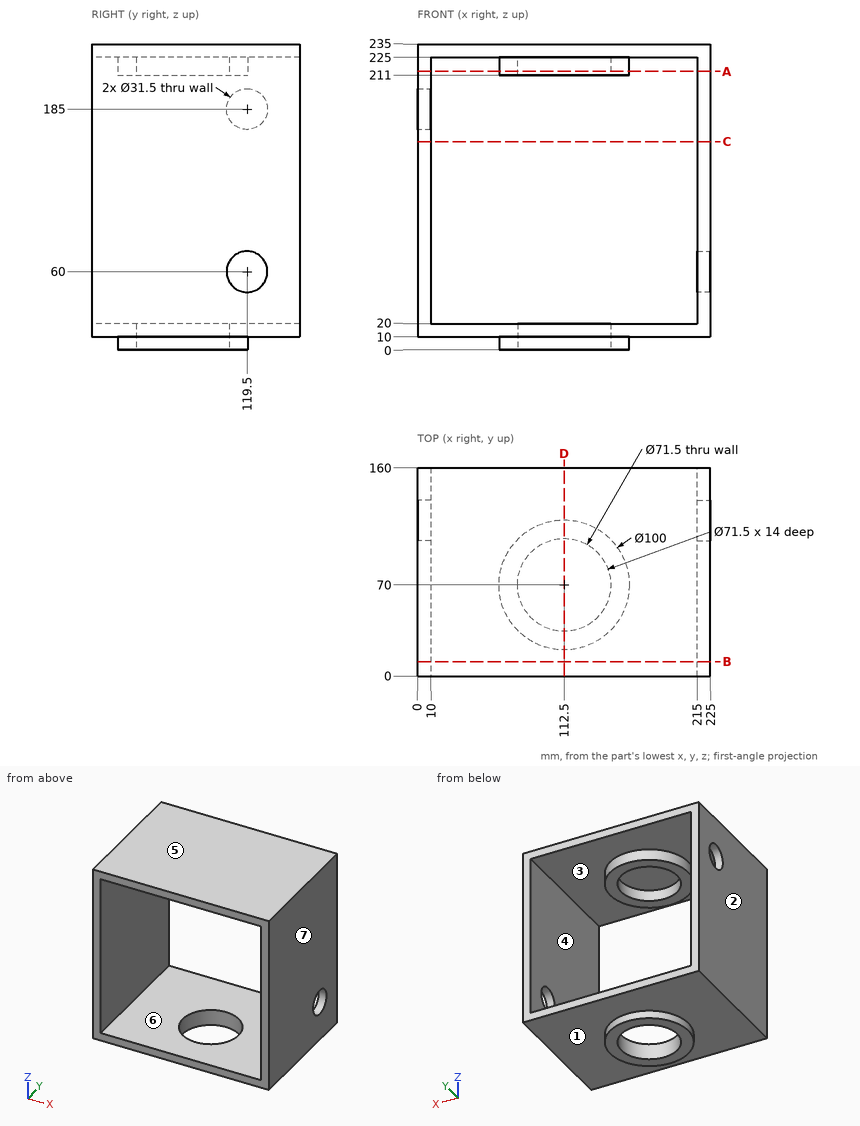
Can you work these out from the drawing? Everything is in mm from the part's minimum corner. A direction names the side the tool comes from. Coordinates: 2 decimals unless noted, no trailing zeros. Loops run counter-clockwise (first coordinate to the right, second up) from the corner with the lowest first, then second, coordinate; pieces in that order, holes last.
1) Imagine slicing it at C-C on z = 160. List the corners of the cut face in (x, y) for me.
2) Imagine slicing it at A-A on z = 214. List the corners of the cut face in (x, y) for me.
3) I need wall thicknesses on probe 1 along X at (y, z) = (85, 62.5); probe 2 along Z at (x, y) = (172, 91.5); probe 3 along Y at (x, z) = (112.5, 216). Which ranges of each line are inside material? Lowest first, please.
4) Imagine slicing it at D-D on x = 112.5. List the corners of the cut face in (y, z) for me.
5) Imagine slicing it at B-B on y = 11. List the corners of the cut face in (x, z) for me.
6) Thinking about a two-plate mould opening in Z: for the marked faces 5, 6 and 7, which applies, pulls with the +Z half, pulls with the -Z half, needs draft (parallel to the pull), parting line crosses it, or undercut?
7) Which directions (+Z, -Z, +X, -X, +Y, -Y) give clear straight access to the entire face, cutting with the end or side of a thin tool? Please do the marked faces 1, 2, 3 and 4.
8) For pin 1 (3 mm diameter, centred on x = 160, y = 66.5, fed in from -Z), with a flat end and sliding along its axis, tell me the tip position at first contact or that it passes through.
Completed:
1. outline: (0, 0) - (10, 0) - (10, 160) - (0, 160) - close; (215, 0) - (225, 0) - (225, 160) - (215, 160) - close
2. outline: (0, 0) - (10, 0) - (10, 160) - (0, 160) - close; circle Ø100 at (112.5, 70); (215, 0) - (225, 0) - (225, 160) - (215, 160) - close; hole circle Ø71.5 at (112.5, 70)
3. probe 1: x = 0 to 10, 215 to 225
3. probe 2: z = 10 to 20, 225 to 235
3. probe 3: y = 20 to 34.25, 105.75 to 120
4. outline: (0, 10) - (20, 10) - (20, 0) - (34.25, 0) - (34.25, 20) - (0, 20) - close; (0, 225) - (20, 225) - (20, 211) - (34.25, 211) - (34.25, 225) - (105.75, 225) - (105.75, 211) - (120, 211) - (120, 225) - (160, 225) - (160, 235) - (0, 235) - close; (105.75, 0) - (120, 0) - (120, 10) - (160, 10) - (160, 20) - (105.75, 20) - close
5. outline: (0, 10) - (225, 10) - (225, 235) - (0, 235) - close; hole (10, 20) - (215, 20) - (215, 225) - (10, 225) - close
6. face 5: pulls with the +Z half
6. face 6: undercut
6. face 7: needs draft
7. face 1: -Z
7. face 2: +Z, -Z, -X, +Y, -Y
7. face 3: none
7. face 4: +Y, -Y
8. pin 1: stops at z = 0
